Check sheet for the modelled part. Datum: model origin and axes. Units: mm. Coordinates: 2 decimals unless noted, no trailing zeros. Loops run counter-clockwise (first coordinate to the right, second up) from the corner with the lowest first, then second, coordinate; pieces in that order, holes last. Notation, with made-up numbers: M -9,-16 L 8,-16 A11 cw 8,-5 Z; hole C -40,-12 d6. An arc over 180 degrees is marked long. Answer in a Markdown table with one row per item. Add a question column.
Autodesk Inventor part; units mm, degrees
ref_plane "YZ Plane" through (0, 0, 0) normal (1, 0, 0) x (0, 1, 0)
ref_plane "XZ Plane" through (0, 0, 0) normal (0, 1, 0) x (-1, 0, 0)
ref_plane "XY Plane" through (0, 0, 0) normal (0, 0, 1) x (1, 0, 0)
sketch "Sketch1" plane through (0, 0, 0) normal (0, 1, 0) x (-1, 0, 0)
  line L0 (0, 0) -> (-800, 0)
  line L1 (-800, 0) -> (-800, -1600)
  line L2 (-800, -1600) -> (0, -1600)
  line L3 (0, -1600) -> (0, 0)
  dimension "d0" = 800
  dimension "d1" = 1600
extrude "Extrusion1" add sketch "Sketch1" along normal blind 26
sketch "Sketch2" plane through (0, 26, 0) normal (0, 1, 0) x (1, 0, 0)
  line L0 (75, 75) -> (725, 75)
  line L1 (725, 75) -> (725, 1525)
  line L2 (725, 1525) -> (75, 1525)
  line L3 (75, 1525) -> (75, 75)
  line L4 (0, 1600) -> (0, 0)
  line L5 (800, 0) -> (800, 1600)
  line L6 (0, 0) -> (800, 0)
  line L7 (800, 1600) -> (0, 1600)
  dimension "d4" = 75
  dimension "d5" = 75
  dimension "d6" = 75
  dimension "d7" = 75
extrude "Extrusion2" add sketch "Sketch2" along normal blind 26 contours L3 L2 L1 L0
sketch "Sketch3" plane through (0, 52, 0) normal (0, 1, 0) x (1, 0, 0)
  point P0 (0, 0)
sketch "Sketch4" plane through (0, 52, 0) normal (0, 1, 0) x (1, 0, 0)
  point P0 (0, 0)
properties part number "tabletop" material "Walnut"
Q1. Cross-section at B-B (z = -1029.5). Record the cut outline in (x, y), plus the area to 3 significant figures.
Q2. Go/stop test with flat-tipped pins: pin 1 (3 mm diameter, centred on x = 544.5, y = 10, fed in from +Z); pin 2 (8 mm diameter, centred on y = 34.5, z = -772.5, fed in from +X); pin 3 (8 mm diameter, centred on x = 481, y = 44.5, fed in from -Z); pin 4 (8 mm diameter, centred on x = 431, y = 42.5, fed in from +Z). Record where each tip stops, or that it passes through.
Q3. Thickness scan on L1, parallel to X at y = 29.5, z = -1191; L2, parallel to Z at x = 694, y = 31.5; L3, parallel to Y at x = 750, z = -387. Record the ranges inside material, lowest first.
Q4. Cross-section at A-A (x = 608.5). Record the cut outline in (y, z).
Answer key:
| question | item | result |
|---|---|---|
| 1 | outline | M 0,0 L 800,0 L 800,26 L 725,26 L 725,52 L 75,52 L 75,26 L 0,26 Z |
| 1 | area | 37,700 mm^2 |
| 2 | pin 1 | z = 0 |
| 2 | pin 2 | x = 725 |
| 2 | pin 3 | z = -1525 |
| 2 | pin 4 | z = -75 |
| 3 | L1 | 75 to 725 |
| 3 | L2 | -1525 to -75 |
| 3 | L3 | 0 to 26 |
| 4 | outline | M 0,-1600 L 26,-1600 L 26,-1525 L 52,-1525 L 52,-75 L 26,-75 L 26,0 L 0,0 Z |
